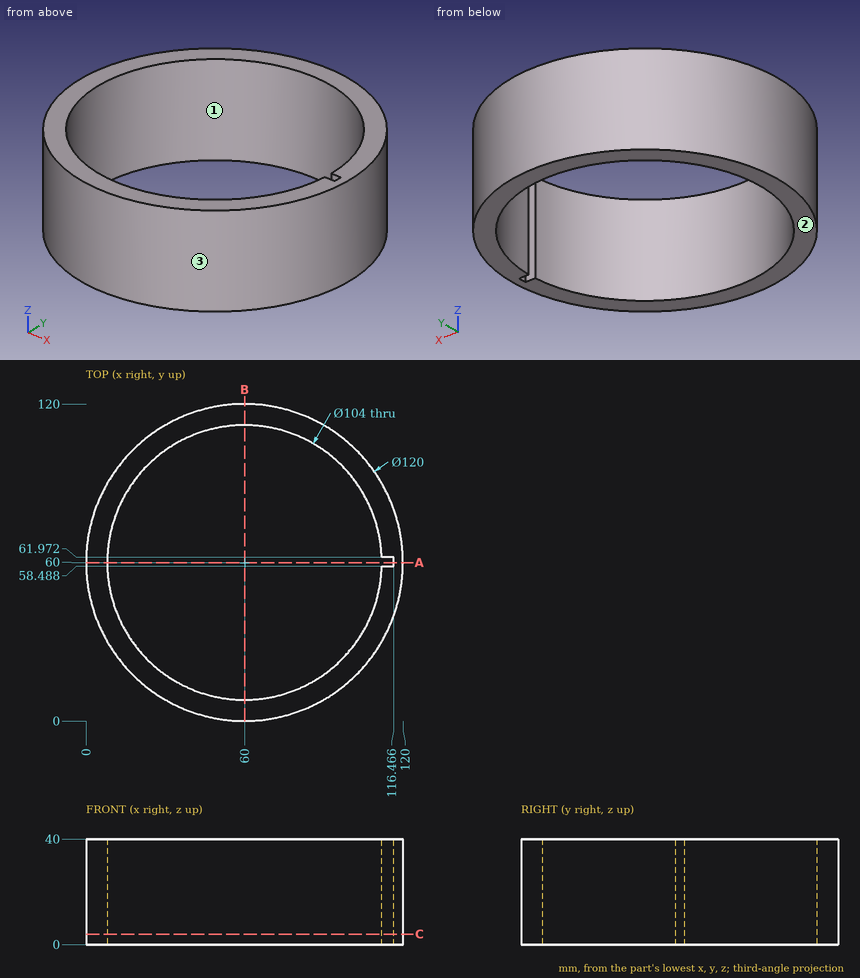
Job drawing, mm, ordinate dimensions from the low corner. One solid piece. Give positions to 0.01 mm unless a question says otherwise; leave off trailing zeros. Order: outer loops, then holes, each group sorted by start corner. A loop starts at its lowest first (then second) coordinate and runs counter-clockwise, first axis right, second up. Notation, with made-up numbers: (-19, -23) - (22, -23) arc R18 ccw to (22, -3) - close; hole circle Ø4 at (81.5, -15.75). An arc over 180 degrees is marked (long way). Answer in a Markdown table with one row per item.
1. Probe probe 1 along Y at (x, z) = (60, 16); probe 2 along Y at (x, z) = (113, 4) (1 decimal); probe 3 along X at (y, z) = (42.5, 30). List the from-to ranges inside material, lowest first. Write a range as [from, to].
Data:
| item | result |
|---|---|
| probe 1 | y = [0, 8], [112, 120] |
| probe 2 | y = [31.9, 58.5], [62, 88.1] |
| probe 3 | x = [2.61, 11.03], [108.97, 117.39] |
2. Saw through at A-A, the plane y = 60. Give the cut face in (x, z) (1 decimal).
Data:
| item | result |
|---|---|
| outline | (0, 0) - (8, 0) - (8, 40) - (0, 40) - close; (116.5, 0) - (120, 0) - (120, 40) - (116.5, 40) - close |
3. Saw through at C-C, the plane z = 4. Give the cut face in (x, y) (1 decimal), plus the area to 3 significant figures.
Data:
| item | result |
|---|---|
| outline | circle Ø120 at (60, 60); hole (112, 58.5) - (116.5, 58.5) - (116.5, 62) - (112, 62) arc R52 ccw (long way) to start |
| area | 2,800 mm² |
4. Saw through at B-B, the plane x = 60. Give the cut face in (y, z), plus the area to 3 significant figures.
Data:
| item | result |
|---|---|
| outline | (0, 0) - (8, 0) - (8, 40) - (0, 40) - close; (112, 0) - (120, 0) - (120, 40) - (112, 40) - close |
| area | 640 mm² |
5. Pull direction X, two halves, no side cores. Call the marked faces 1, 2 and 3: pulls with the +X half, pulls with the -X half, needs draft (parallel to the pull), parting line crosses it, or undercut.
Data:
| item | result |
|---|---|
| face 1 | undercut |
| face 2 | needs draft |
| face 3 | parting line crosses it |
6. Flat gauge pins, fed straight in: pin 1 (3 mm diameter, centred on y = 103, z = 27, fed in from -X); pin 2 (5 mm diameter, centred on x = 79.5, z = 8.5, fed in from +Y); pin 3 (1.5 mm diameter, centred on y = 60.5, z = 4, fed in from -X); pin 4 (3.5 mm diameter, centred on x = 115, z = 20, fed in from -Y). Where does each tip first touch, or does it go through?
Data:
| item | result |
|---|---|
| pin 1 | stops at x = 16.67 |
| pin 2 | stops at y = 117.54 |
| pin 3 | stops at x = 0 |
| pin 4 | stops at y = 32.35 |
